from build123d import *

# Parameters (mm, degrees)
SKETCH_1_W          = 62
SKETCH_1_H          = 32
EXTRUDE_1_DEPTH     = 8
SKETCH_2_R          = 7
EXTRUDE_2_DEPTH     = 10
SKETCH_6_W          = 21.388804526
SKETCH_6_H          = 8.444348029
CUT_EXTRUDE_1_DEPTH = 42.243181422


with BuildPart() as part:
    # 草图1 → 凸台-拉伸1 (new body)
    with BuildSketch(Plane(origin=(0, 0, 0), x_dir=(1, 0, 0), z_dir=(0, 1, 0))):
        Rectangle(SKETCH_1_W, SKETCH_1_H)
    extrude(amount=EXTRUDE_1_DEPTH)

    # 草图2 → 凸台-拉伸2 (add)
    with BuildSketch(Plane(origin=(0, 0, -16), x_dir=(-1, 0, 0), z_dir=(0, 0, -1))):
        with BuildLine():
            Line((-24, 21), (-24, 8))
            Line((-24, 8), (31, 8))
            Line((31, 8), (31, 34))
            Line((31, 34), (-11, 34))
            ThreePointArc((-11, 34), (-20.192388155, 30.192388155), (-24, 21))
        make_face()
        with Locations((-11, 21)):
            Circle(SKETCH_2_R, mode=Mode.SUBTRACT)
    extrude(amount=-EXTRUDE_2_DEPTH)

    # 草图5 → 放样1 section 0
    with BuildSketch(Plane(origin=(0, 8, 0), x_dir=(1, 0, 0), z_dir=(0, 1, 0))):
        with BuildLine():
            Line((-3, -16), (-3, 6))
            Line((-3, 6), (-31, 6))
            Line((-31, 6), (-31, -16))
            Line((-31, -16), (-3, -16))
        make_face()
    # 草图4 → 放样1 section 1
    with BuildSketch(Plane(origin=(0, 34, 0), x_dir=(1, 0, 0), z_dir=(0, 1, 0))):
        with BuildLine():
            Line((-31, 6), (-31, 0))
            Line((-31, 0), (-17, 0))
            Line((-17, 0), (-17, 6))
            Line((-17, 6), (-31, 6))
        make_face()
    loft()

    # 草图6 → 切除-拉伸1 (cut, through all)
    with BuildSketch(Plane(origin=(0, 22, 0), x_dir=(1, 0, 0), z_dir=(0, 1, 0))):
        with Locations((-20.305597737, -4.222174015)):
            Rectangle(SKETCH_6_W, SKETCH_6_H)
    extrude(amount=CUT_EXTRUDE_1_DEPTH, mode=Mode.SUBTRACT)


solid = part.part
Here's how the part is built. I have some questions about the finished solid (model axes, mm). A direction names the side the tool comes from. Round coordinates to 2 decimals unless told otherwise and drop trailing zeros. Write each loop counter-clockwise with the first axis right and the second up, starting at its lowest first coordinate (ties: lowest second). Pieces come first, ordered by that corner, then holes.
1. For faces 1 (the flat face through (0, 4, 16)), 2 (the flat face through (-23, 28, 0)), which set-ups out of +Z, -Z, +X, -X, +Y, -Y let a thin tool reach every point of the face, with its end or its side?
2. Will these pins go through, and if not, where does the flat tip stop? pin 1 Ø8 at (y, z) = (17.5, -11) entering from +X; pin 2 Ø1.5 at (x, z) = (-17.5, 8.5) entering from +Y; pin 3 Ø1.5 at (x, y) = (-7.5, 9.5) entering from +Z; pin 4 Ø11 at (x, y) = (11, 21) entering from +Z.
3. Suppose I cut it at C-C (x = 20). List the corners of the cut face in (y, z) for me.
4. If we mould it in two halves opening along X, with no side actions, what happens to faces 3 (the cylindrical face through (12.517, 14.166, -11.07)), 4 (the flat face through (3.8, 21.2, -6)), 5 (the flat face through (-31, 17, -2)), 6 (the flat face through (24, 15, -11))? For each: released by +X, released by -X, zero draft, split by the parting line, or undercut.
5. Suppose I cut it at D-D (x = 26.5). List the corners of the cut face in (y, z) for me, and give its area (3 significant figures).
6. I need wall thicknesses on L1, parallel to Y at x = 11, z = -11; L2, parallel to Z at x = 5, y = 27; L3, parallel to Y at x = 3.5, z = 14.5. Which ranges of each line are inside material? Lowest first, please.
7. Suppose I cut it at B-B (x = 2.5). List the corners of the cut face in (y, z) for me, and give its area (3 significant figures).
8. Suppose I cut it at A-A (z = -7). List the corners of the cut face in (x, y) for me.
Answer sheet:
1. face 1: +Z, +X, -X, +Y, -Y
1. face 2: +Z, +X, -X, +Y
2. pin 1: stops at x = 24
2. pin 2: stops at y = 21.41
2. pin 3: stops at z = 15.54
2. pin 4: passes through
3. outline: (0, -16) - (30.38, -16) - (30.38, -6) - (8, -6) - (8, 16) - (0, 16) - close
4. face 3: undercut
4. face 4: zero draft
4. face 5: released by -X
4. face 6: released by +X
5. outline: (0, -16) - (8, -16) - (8, 16) - (0, 16) - close
5. area: 256 mm2
6. L1: y = 0 to 14, 28 to 34
6. L2: z = -16 to -6
6. L3: y = 0 to 8
7. outline: (0, -16) - (34, -16) - (34, -6) - (8, -6) - (8, 16) - (0, 16) - close
7. area: 516 mm2
8. outline: (-31, 0) - (31, 0) - (31, 8) - (24, 8) - (24, 21) arc R13 ccw to (11, 34) - (-31, 34) - close; hole circle Ø14 at (11, 21)
